The listing builds one solid part. Answer for the finished solid, in the listing's coordinates (mm). A direction names the side the tool comes from. Give positions to 0.01 mm unless a question says otherwise; leave off trailing zeros. Return JSON: item names as keys, results as strings.
from build123d import *

# Parameters (mm, degrees)
SKETCH1_W                  = 298.45
SKETCH1_H                  = 495.3
BOSS_EXTRUDE1_DEPTH        = 4.7625
CUT_EXTRUDE1_DEPTH         = 290.291114191
CUT_EXTRUDE1_DEPTH_BACK    = 290.291114191
SKETCH3_W                  = 196.85
SKETCH3_H                  = 114.3
SKETCH20_W                 = 47.879
SKETCH20_H                 = 47.879
CUT_EXTRUDE5_DEPTH         = 290.291114191
F_10_CLEARANCE_HOLE1_D     = 5.1054
F_10_CLEARANCE_HOLE1_DEPTH = 10.668
F_10_CLEARANCE_HOLE1_TIP   = 1.533816902
F_10_CLEARANCE_HOLE4_D     = 5.1054
LPATTERN3_COUNT            = 3
LPATTERN3_PITCH            = 63.5
MIRROR2_COPY_1_D           = 5.1054
MIRROR2_COPY_2_D           = 5.1054
F_10_CLEARANCE_HOLE5_D     = 5.1054
LPATTERN4_COUNT            = 3
LPATTERN4_PITCH            = 96.52
LPATTERN4_COL_COUNT        = 3
LPATTERN4_COL_PITCH        = 96.52
MIRROR3_COPY_1_D           = 5.1054
MIRROR3_COPY_2_D           = 5.1054
MIRROR3_COPY_3_D           = 5.1054
MIRROR3_COPY_4_D           = 5.1054
F_10_CLEARANCE_HOLE6_D     = 5.1054


with BuildPart() as part:
    # Sketch1 → Boss-Extrude1 (new, symmetric)
    with BuildSketch(Plane(origin=(0, 0, 0), x_dir=(1, 0, 0), z_dir=(0, 1, 0))):
        Rectangle(SKETCH1_W, SKETCH1_H)
    extrude(amount=BOSS_EXTRUDE1_DEPTH, both=True)

    # Sketch3 → Cut-Extrude1 (cut, two sides: drawn at the far end of the back side and taken through both)
    with BuildSketch(Plane(origin=(0, 4.7625, 0), x_dir=(1, 0, 0), z_dir=(0, 1, 0)).offset(-CUT_EXTRUDE1_DEPTH_BACK)):
        with Locations((0, -44.45)):
            Rectangle(SKETCH3_W, SKETCH3_H)
    extrude(amount=CUT_EXTRUDE1_DEPTH + CUT_EXTRUDE1_DEPTH_BACK, mode=Mode.SUBTRACT)

    # Sketch20 → Cut-Extrude5 (cut, through all)
    with BuildSketch(Plane.XZ.offset(4.7625)):
        with Locations((0, 171.45)):
            Rectangle(SKETCH20_W, SKETCH20_H)
    extrude(amount=-CUT_EXTRUDE5_DEPTH, mode=Mode.SUBTRACT)

    # #10 Clearance Hole1
    with Locations(Plane(origin=(0, -4.7625, 0), x_dir=(-1, 0, 0), z_dir=(0, -1, 0))):
        with Locations((-38.1, -155.575), (38.1, -155.575), (38.1, -187.325), (-38.1, -187.325)):
            Hole(F_10_CLEARANCE_HOLE1_D / 2, depth=F_10_CLEARANCE_HOLE1_DEPTH)
            with Locations((0, 0, -(F_10_CLEARANCE_HOLE1_DEPTH + F_10_CLEARANCE_HOLE1_TIP / 2))):  # 118° drill point
                Cone(0, F_10_CLEARANCE_HOLE1_D / 2, F_10_CLEARANCE_HOLE1_TIP, mode=Mode.SUBTRACT)

    # #10 Clearance Hole4 (through all)
    with Locations(Plane(origin=(0, 4.7625, 0), x_dir=(1, 0, 0), z_dir=(0, 1, 0))):
        with Locations((-63.5, 241.3)):
            f_10_clearance_hole4 = Hole(F_10_CLEARANCE_HOLE4_D / 2)

    # LPattern3: #10 Clearance Hole4 ×3
    with Locations(*[(i * LPATTERN3_PITCH, 0, 0) for i in range(1, LPATTERN3_COUNT)]):
        add(f_10_clearance_hole4, mode=Mode.SUBTRACT)

    # Mirror2: #10 Clearance Hole4 across plane
    add(f_10_clearance_hole4.mirror(Plane.XY), mode=Mode.SUBTRACT)

    # Mirror2 copy 1 (through all)
    with Locations(Plane(origin=(63.5, 4.7625, 0), x_dir=(1, 0, 0), z_dir=(0, 1, 0))):
        with Locations((-63.5, -241.3)):
            Hole(MIRROR2_COPY_1_D / 2)

    # Mirror2 copy 2 (through all)
    with Locations(Plane(origin=(127, 4.7625, 0), x_dir=(1, 0, 0), z_dir=(0, 1, 0))):
        with Locations((-63.5, -241.3)):
            Hole(MIRROR2_COPY_2_D / 2)

    # #10 Clearance Hole5 (through all)
    with Locations(Plane(origin=(0, 4.7625, 0), x_dir=(1, 0, 0), z_dir=(0, 1, 0))):
        with Locations((-142.875, 0)):
            f_10_clearance_hole5 = Hole(F_10_CLEARANCE_HOLE5_D / 2)

    # LPattern4: #10 Clearance Hole5 ×3
    with Locations(*[(0, 0, -i * LPATTERN4_PITCH) for i in range(1, LPATTERN4_COUNT)]):
        add(f_10_clearance_hole5, mode=Mode.SUBTRACT)

    # LPattern4 col: #10 Clearance Hole5 ×3
    with Locations(*[(0, 0, i * LPATTERN4_COL_PITCH) for i in range(1, LPATTERN4_COL_COUNT)]):
        add(f_10_clearance_hole5, mode=Mode.SUBTRACT)

    # Mirror3: #10 Clearance Hole5 across plane
    add(f_10_clearance_hole5.mirror(Plane(origin=(0, 0, 0), x_dir=(0, 0, 1), z_dir=(1, 0, 0))), mode=Mode.SUBTRACT)

    # Mirror3 copy 1 (through all)
    with Locations(Plane(origin=(0, 4.7625, -96.52), x_dir=(-1, 0, 0), z_dir=(0, 1, 0))):
        with Locations((-142.875, 0)):
            Hole(MIRROR3_COPY_1_D / 2)

    # Mirror3 copy 2 (through all)
    with Locations(Plane(origin=(0, 4.7625, -193.04), x_dir=(-1, 0, 0), z_dir=(0, 1, 0))):
        with Locations((-142.875, 0)):
            Hole(MIRROR3_COPY_2_D / 2)

    # Mirror3 copy 3 (through all)
    with Locations(Plane(origin=(0, 4.7625, 96.52), x_dir=(-1, 0, 0), z_dir=(0, 1, 0))):
        with Locations((-142.875, 0)):
            Hole(MIRROR3_COPY_3_D / 2)

    # Mirror3 copy 4 (through all)
    with Locations(Plane(origin=(0, 4.7625, 193.04), x_dir=(-1, 0, 0), z_dir=(0, 1, 0))):
        with Locations((-142.875, 0)):
            Hole(MIRROR3_COPY_4_D / 2)

    # #10 Clearance Hole6 (through all)
    with Locations(Plane(origin=(0, 4.7625, 0), x_dir=(1, 0, 0), z_dir=(0, 1, 0))):
        with Locations((120.65, 39.4255), (120.65, -128.3255), (-120.65, -128.3255), (-120.65, 39.4255)):
            Hole(F_10_CLEARANCE_HOLE6_D / 2)


solid = part.part
(1) The part is cut by section A-A (y = 0). Give the number of separate pieces and of enclosed holes in the cut face, and give its area (3 significant figures).
Values follow:
{"separate pieces": "1", "enclosed holes": "26", "area": "123,000 mm²"}
(2) Determine the mould class of faces 3 (the flat face through (149.225, 0, 3)), 4 (the flat face through (-23.94, 0, 171)), 5 (the flat face through (-2, 0, 247.65)) for opening direction Z: released by +Z, released by -Z, zero draft, split by the parting line, or undercut.
Values follow:
{"face 3": "zero draft", "face 4": "undercut", "face 5": "released by +Z"}
(3) A tool of negligible diameter and unlimited length cuts with its end or side. For faces 1 (the flat face through (-98.425, 0, 45)), 2 (the flat face through (-2, 4.762, -59)), from which of +Z, -Z, +X, -X, +Y, -Y can it reach the whole face along a straight path? Write none if from no direction.
Values follow:
{"face 1": "+Y, -Y", "face 2": "+Z, -Z, +X, -X, +Y"}
(4) Straight lines are drawn through the part: line 1 along Z through (x, y) = (-13.5, -1.5); line 2 along X through (y, z) = (-1.25, 193.04) (1 decimal); line 3 along Z through (x, y) = (-52, 0). For each, find the intervals that lie inside material, in ascending order.
Values follow:
{"line 1": "-247.65 to -12.7, 101.6 to 147.51, 195.39 to 247.65", "line 2": "-149.2 to -145.4, -140.3 to -23.9, 23.9 to 140.3, 145.4 to 149.2", "line 3": "-247.65 to -12.7, 101.6 to 247.65"}
